Verification items for the finished model (mm, model axes). A direction names the side the tool comes from. Round coordinates to 2 decimals unless told otherwise and drop trailing zeros. Order: outer loops, then holes, each group sorted by start corner. A loop starts at its lowest first (then second) coordinate and runs counter-clockwise, first axis right, second up. Notation, with made-up numbers: M 15,87 L 55,87 A17 ccw 55,114 Z; hole C -35.5,50 d10. An arc over 180 degrees is marked long. Return JSON: item names as keys, results as strings. Group by question number.
from build123d import *

# Parameters (mm, degrees)
SKETCH1_W                  = 36
SKETCH1_H                  = 36
BOSS_EXTRUDE1_DEPTH        = 1.6
F_3_2_3_2_DIAMETER_HOLE1_D = 3.25
BOSS_EXTRUDE2_DEPTH        = 4.65
SKETCH5_R                  = 14.2
BOSS_EXTRUDE3_DEPTH        = 7.8
SKETCH6_R                  = 15
BOSS_EXTRUDE4_DEPTH        = 8
SKETCH7_R                  = 14
BOSS_EXTRUDE5_DEPTH        = 9.5
SKETCH8_W                  = 21
SKETCH8_H                  = 5.5
BOSS_EXTRUDE6_DEPTH        = 2.5


with BuildPart() as part:
    # Sketch1 → Boss-Extrude1 (new body)
    with BuildSketch(Plane(origin=(0, 0, 0), x_dir=(1, 0, 0), z_dir=(0, 1, 0))):
        Rectangle(SKETCH1_W, SKETCH1_H)
    extrude(amount=BOSS_EXTRUDE1_DEPTH)

    # Ø3.2 (3.2) Diameter Hole1 (through all)
    with Locations(Plane(origin=(0, 1.6, 0), x_dir=(1, 0, 0), z_dir=(0, 1, 0))):
        with Locations((-14.25, 14.25), (14.25, 14.25), (14.25, -14.25), (-14.25, -14.25)):
            Hole(F_3_2_3_2_DIAMETER_HOLE1_D / 2)

    # Sketch4 → Boss-Extrude2 (add)
    with BuildSketch(Plane(origin=(0, 1.6, 0), x_dir=(1, 0, 0), z_dir=(0, 1, 0))):
        with BuildLine():
            Line((-8.125, -8.125), (8.125, -8.125))
            Line((8.125, -8.125), (8.125, -1.9))
            Line((8.125, -1.9), (9.5, -1.9))
            ThreePointArc((9.5, -1.9), (11.4, 0), (9.5, 1.9))
            Line((9.5, 1.9), (8.125, 1.9))
            Line((8.125, 1.9), (8.125, 8.125))
            Line((8.125, 8.125), (-8.125, 8.125))
            Line((-8.125, 8.125), (-8.125, 1.9))
            Line((-8.125, 1.9), (-9.5, 1.9))
            ThreePointArc((-9.5, 1.9), (-11.4, 0), (-9.5, -1.9))
            Line((-9.5, -1.9), (-8.125, -1.9))
            Line((-8.125, -1.9), (-8.125, -8.125))
        make_face()
    extrude(amount=BOSS_EXTRUDE2_DEPTH)

    # Sketch5 → Boss-Extrude3 (add)
    with BuildSketch(Plane(origin=(0, 6.25, 0), x_dir=(1, 0, 0), z_dir=(0, 1, 0))):
        with Locations(Location((0, 0, 0), (0, 0, 270))):
            Circle(SKETCH5_R)
    extrude(amount=BOSS_EXTRUDE3_DEPTH)

    # Sketch6 → Boss-Extrude4 (add)
    with BuildSketch(Plane(origin=(0, 14.05, 0), x_dir=(1, 0, 0), z_dir=(0, 1, 0))):
        with Locations(Location((0, 0, 0), (0, 0, 270))):
            Circle(SKETCH6_R)
    extrude(amount=BOSS_EXTRUDE4_DEPTH)

    # Sketch7 → Boss-Extrude5 (add)
    with BuildSketch(Plane(origin=(0, 22.05, 0), x_dir=(1, 0, 0), z_dir=(0, 1, 0))):
        with Locations(Location((0, 0, 0), (0, 0, 270))):
            Circle(SKETCH7_R)
    extrude(amount=BOSS_EXTRUDE5_DEPTH)

    # Sketch8 → Boss-Extrude6 (add)
    with BuildSketch(Plane.XZ):
        with Locations((0, 14.25)):
            Rectangle(SKETCH8_W, SKETCH8_H)
    extrude(amount=BOSS_EXTRUDE6_DEPTH)

    # Sketch9 → Cut-Revolve1 (revolve, cut)
    with BuildSketch(Plane.XY, mode=Mode.PRIVATE) as cut_revolve1_sk:
        Polygon((0, 31.55), (0, 26.55), (7, 26.55), (10.85, 30.55), (12.35, 30.55), (12.35, 31.55), align=None)
    revolve(cut_revolve1_sk.sketch.rotate(Axis((0, 31.55, 0), (0, -1, 0)), 180), axis=Axis((0, 31.55, 0), (0, -1, 0)), mode=Mode.SUBTRACT)


solid = part.part
1. Access from +Z, -Z, +X, -X, +Y, -Y to the whole of each face (thin tool, end or side, straight path). Record for faces 4 (the face through (0, -1, 11.5)), 5 (the face through (0, 6.25, 9)), 6 (the face through (0, 30.55, 11)), 7 (the face through (-8.125, 4, -5)).
2. Go/stop test with flat-tipped pins: pin 1 (3 mm diameter, centred on y = 10, z = 0, fed in from +X); pin 2 (15 mm diameter, centred on x = 0, z = 0, fed in from +Y); pin 3 (8 mm diameter, centred on y = 9, z = 11.5, fed in from -X). Record where each tip stops, or that it passes through.
3. Cross-section at C-C (y = 12.5). Enter the section's corners in (x, z).
4. Thickness scan on line 1 along Z through (x, y) = (-14.25, 1.25) (3 decimals); line 2 along Y through (x, z) = (5, 2.5). Record the ranges inside material, lowest first. Write a range as from..to.
5. Draft check along Y on faces 1 (the face through (0, 26.55, 0)), 2 (the face through (-11.4, 3.9, 0)), 3 (the face through (0, 1, 18)). Enter one of: +Y half, -Y half, draft (parallel to the pull), parting line (faces both ways), or undercut.
6. Cross-section at B-B (y = 24). Enter the section's corners in (x, z), plus the area to 3 significant figures.
Computed:
{
 "1": {"face 4": "-Z, +X, -X, -Y", "face 5": "none", "face 6": "+Y", "face 7": "-Z, -X"},
 "2": {"pin 1": "stops at x = 14.2", "pin 2": "stops at y = 27.07", "pin 3": "stops at x = -12.06"},
 "3": {"outline": "C 0,0 d28.4"},
 "4": {"line 1": "z = -18..-15.875, -12.625..12.625, 15.875..18", "line 2": "y = 0..26.55"},
 "5": {"face 1": "+Y half", "face 2": "undercut", "face 3": "draft"},
 "6": {"outline": "C 0,0 d28", "area": "616 mm²"}
}
